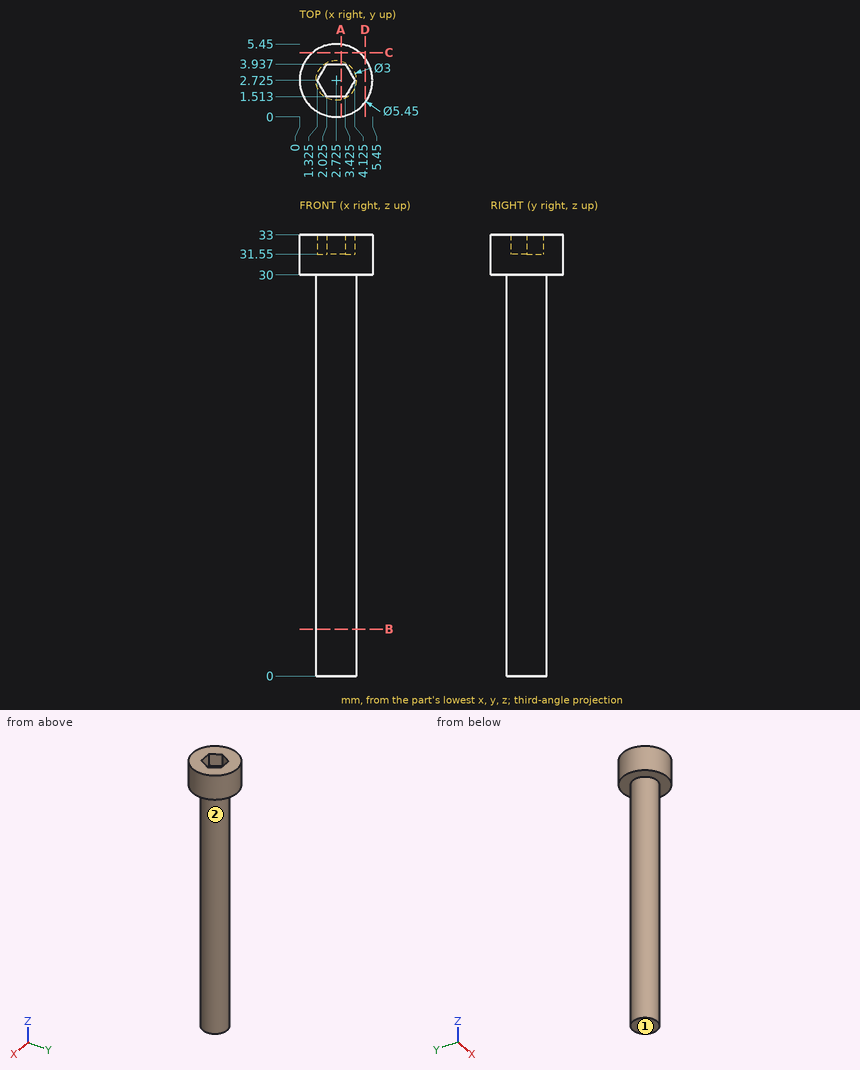
Input: dimensioned drawing with shaded views. Units: mm. Origin: part minimum x, y, z. A direction names the side the tool comes from. Round coordinates to 2 decimals unless told otherwise and drop trailing zeros. Loops run counter-clockwise (first coordinate to the right, second up) from the corner with the lowest first, then second, coordinate; pieces in that order, holes last. Notation, with made-up numbers: (-24.5, 39) -> (30.5, 39) arc R26 ccw to (30.5, 62) -> close; hole circle Ø1 at (0.25, 61). An arc over 180 degrees is marked (long way). Answer as a JSON object with one key per item and string values. Group by question number.
Q1. Section query A-A (x = 3.1). Output: boundary loops of the cut face in (y, z).
Q2. Section query B-B (z = 3.5). Output: boundary loops of the cut face in (x, y) (1 decimal).
Q3. Access query for the marked faces 1 and 2. Directions: +Z, -Z, +X, -X, +Y, -Y. A direction counts if a zero-diameter tool reaches every point of the face in a straight line with its end or side. Return the directions, or none.
Q4. Section query D-D (x = 4.9). Output: boundary loops of the cut face in (y, z).
Q5. Contact query for flat-ended pins moving along their axis: P1, Ø1, axis at y = 3, z = 16.5, coming from the -X side (3 decimals); P2, Ø1.5, axis at x = 3, z = 25.5, coming from the +Y side (3 decimals); P3, Ø1.5, axis at x = 4.5, z = 25, coming from the -Y side. Output: stop coordinate, or through.
Q6. Section query C-C (y = 4.8). Output: boundary loops of the cut face in (x, z), plus the area to 3 significant figures.
Q7. Ray query, line 1 (Y direction, x = 2.7, z = 8) (1 decimal); line 2 (Z direction, x = 3.6, y = 0.35); line 3 (Y direction, x = 3.25, z = 12). Return the intervals inside material, ascending. Write a range as from..to.
Completed:
{
 "1": {"outline": "(0.03, 30) -> (1.27, 30) -> (1.27, 0) -> (4.18, 0) -> (4.18, 30) -> (5.42, 30) -> (5.42, 33) -> (3.94, 33) -> (3.94, 31.55) -> (1.51, 31.55) -> (1.51, 33) -> (0.03, 33) -> close"},
 "2": {"outline": "circle Ø3 at (2.7, 2.7)"},
 "3": {"face 1": "-Z, +X, -X, +Y, -Y", "face 2": "-Z"},
 "4": {"outline": "(1.08, 30) -> (4.37, 30) -> (4.37, 33) -> (1.08, 33) -> close"},
 "5": {"P1": "x = 1.225", "P2": "y = 4.225", "P3": "y = 1.63"},
 "6": {"outline": "(0.96, 30) -> (4.49, 30) -> (4.49, 33) -> (0.96, 33) -> close", "area": "10.6 mm²"},
 "7": {"line 1": "1.2..4.2", "line 2": "30..33", "line 3": "1.32..4.13"}
}
